Work out the finished part from the listing and answer in its coordinate system (mm). A direction names the side the tool comes from. Round coordinates to 2 decimals unless told otherwise and drop trailing zeros. Order: outer loops, then holes, each group sorted by start corner. A loop starts at its lowest first (then second) coordinate and runs counter-clockwise, first axis right, second up. Notation, with made-up numbers: (63, -29) - (76, -29) arc R28 ccw to (76, 5) - close; hole circle Ø10 at (45, -40). An arc over 180 degrees is marked (long way). One line per question, with ' | ' between items. Start each with the question number.
from build123d import *

# Parameters (mm, degrees)
FILETE1_R             = 0.5
CORTE_EXTRUS_O1_DEPTH = 6.5
FILETE2_R             = 0.3
CHANFRO1_SIZE         = 0.75


with BuildPart() as part:
    # Esboço1 → Revolução1 (revolve)
    with BuildSketch(Plane.XY, mode=Mode.PRIVATE) as revolu_o1_sk:
        Polygon((0, 17.056706853), (9.75, 17.056706853), (9.75, 14.756706853), (7.25, 14.756706853), (7.25, 0.756706853), (5, 0.756706853), (5, -9.243293147), (4.75, -9.243293147), (4.75, -24.243293147), (0, -24.243293147), align=None)
    revolve(revolu_o1_sk.sketch.rotate(Axis((0, -39.808803987, 0), (0, 1, 0)), 90), axis=Axis((0, -39.808803987, 0), (0, 1, 0)))

    # Filete1
    filete1_edges = [part.edges().sort_by_distance(p)[0] for p in [
        (0, 14.756706853, 9.75),
        (0, 17.056706853, 9.75),
    ]]
    fillet(filete1_edges, radius=FILETE1_R)

    # Esboço2 → Corte-extrusão1 (cut)
    with BuildSketch(Plane(origin=(0, 17.056706853, 0), x_dir=(1, 0, 0), z_dir=(0, 1, 0))):
        Polygon((0, 4.618802154), (-4, 2.309401077), (-4, -2.309401077), (0, -4.618802154), (4, -2.309401077), (4, 2.309401077), align=None)
    extrude(amount=-CORTE_EXTRUS_O1_DEPTH, mode=Mode.SUBTRACT)

    # Filete2
    filete2_edges = [part.edges().sort_by_distance(p)[0] for p in [
        (2, 10.556706853, -3.464101615),
        (0, 13.806706853, -4.618802154),
        (4, 10.556706853, 0),
        (4, 13.806706853, -2.309401077),
        (2, 10.556706853, 3.464101615),
        (4, 13.806706853, 2.309401077),
        (-2, 10.556706853, 3.464101615),
        (0, 13.806706853, 4.618802154),
        (-4, 10.556706853, 0),
        (-4, 13.806706853, 2.309401077),
        (-2, 10.556706853, -3.464101615),
        (-4, 13.806706853, -2.309401077),
        (2, 17.056706853, -3.464101615),
        (-2, 17.056706853, -3.464101615),
        (-4, 17.056706853, 0),
        (-2, 17.056706853, 3.464101615),
        (2, 17.056706853, 3.464101615),
        (4, 17.056706853, 0),
    ]]
    fillet(filete2_edges, radius=FILETE2_R)

    # Chanfro1
    chanfro1_edges = [part.edges().sort_by_distance(p)[0] for p in [
        (0, -24.243293147, 4.75),
    ]]
    chamfer(chanfro1_edges, length=CHANFRO1_SIZE)


solid = part.part
1) Straight lines are drawn through the part: line 1 (Y direction, x = -4.25, z = 6.5); line 2 (Y direction, x = 2, z = -4.75); line 3 (X direction, y = 4, z = 0). For each, find the intervals that lie inside material, in ascending order.
2) For faces 5 (the flat face through (-1.97, 13.85, -3.48)), 6 (the cylindrical face through (4.637, -16.468, 1.03)), determine the directions among +Z, -Z, +X, -X, +Y, -Y from which every point of the face is accessible in a straight line to the end or side of a thin tool.
3) Determine the mould class of faces 1 (the flat face through (2, 17.057, 4)), 2 (the cylindrical face through (-2.071, 16.971, -3.527)), 3 (the cylindrical face through (-9.667, 15.898, 1.269)), 4 (the cylindrical face through (2.071, 16.971, 3.527)) for opening direction Z: released by +Z, released by -Z, zero draft, split by the parting line, or undercut.
4) Section C-C on y = 4 is taken. Give the vertices of the cut face in (x, z).
5) Section B-B on y = -22 is taken. Give the vertices of the cut face in (x, z), and give its area (3 significant figures).
6) Flat-ended cylindrical pins translate along their axes: pin 1 (10 mm diameter, centred on y = 0, z = -1, fed in from -X); pin 2 (8 mm diameter, centred on y = -13.5, z = 0, fed in from +X); pin 3 (10 mm diameter, centred on x = -7.5, y = -5, fed in from -Z). Find the tip coordinate at first contact, or state that the pin passes through.
Recorded:
1) line 1: y = 14.76 to 17.06 | line 2: y = 0.76 to 17.06 | line 3: x = -7.25 to 7.25
2) face 5: +Y | face 6: -Y
3) face 1: zero draft | face 2: undercut | face 3: split by the parting line | face 4: undercut
4) outline: circle Ø14.5 at (0, 0)
5) outline: circle Ø9.5 at (0, 0) | area: 70.9 mm²
6) pin 1: stops at x = -7.25 | pin 2: stops at x = 4.75 | pin 3: stops at z = -4.33
